from build123d import *

# Parameters (mm, degrees)
F0_R     = 47.5
F0_R_2   = 1
F1_DEPTH = 3.175


with BuildPart() as f1:
    # F0 (on Top) → F1 (new body)
    with BuildSketch(Plane.XY):
        Circle(F0_R)
        with BuildLine():
            ThreePointArc((-30.8198051534, -31.8198051534), (-32.7436846859, -32.2024885858), (-31.1126983722, -31.1126983722))
            ThreePointArc((-31.1126983722, -31.1126983722), (-30.8959256209, -31.437121721), (-30.8198051534, -31.8198051534))
        make_face(mode=Mode.SUBTRACT)
        with Locations((31.8198051534, -31.8198051534)):
            Circle(F0_R_2, mode=Mode.SUBTRACT)
        with Locations((-31.8198051534, 31.8198051534)):
            Circle(F0_R_2, mode=Mode.SUBTRACT)
        with BuildLine():
            ThreePointArc((33.3518936085, -22.0828257415), (4.0043327396, -39.7990617893), (-28.2842712475, -28.2842712475))
            ThreePointArc((-28.2842712475, -28.2842712475), (-30.9736773104, -25.3106956418), (-33.3518936085, -22.0828257415))
            ThreePointArc((-33.3518936085, -22.0828257415), (-35.0740288533, -20.25), (-35.8002348837, -17.8421742585))
            ThreePointArc((-35.8002348837, -17.8421742585), (-34.6410161514, 20), (-2.4483412752, 39.925))
            ThreePointArc((-2.4483412752, 39.925), (0, 40.5), (2.4483412752, 39.925))
            ThreePointArc((2.4483412752, 39.925), (29.1370352902, 27.4049844827), (40, 0))
            ThreePointArc((40, 0), (38.9359049936, -9.1648951072), (35.8002348837, -17.8421742585))
            ThreePointArc((35.8002348837, -17.8421742585), (35.0740288533, -20.25), (33.3518936085, -22.0828257415))
        make_face(mode=Mode.SUBTRACT)
        with Locations((31.8198051534, 31.8198051534)):
            Circle(F0_R_2, mode=Mode.SUBTRACT)
    extrude(amount=F1_DEPTH)


solid = f1.part
Design review of the part built by this model. Coordinates are the model's own, in mm. A direction names the side the tool comes from. Coordinates: 2 decimals unless noted, no trailing zeros. Order: outer loops, then holes, each group sorted by start corner. A loop starts at its lowest first (then second) coordinate and runs counter-clockwise, first axis right, second up.
Item 1: For faces 1 (the cylindrical face through (-35.056, -20.281, 1.565)), 2 (the flat face through (-11, 39, 0)), list the 3-axis set-ups (+Z, -Z, +X, -X, +Y, -Y) from which the entire face can be reached by the end or side of a thin tool; tool diameter is ignored.
Item 2: For pin 1 Ø1.5 at (x, z) = (11.5, 2) entering from -Y; pin 2 Ø1.5 at (y, z) = (6.5, 0.5) entering from -X; pin 3 Ø1.2 at (x, y) = (31.82, -31.82) entering from -Z; pin 4 Ø1.5 at (y, z) = (-33, 1.5) entering from +X, all flat-tipped, find the tip position at first contact; note any pin that passes through.
Item 3: Take a section at B-B, the plane y = 15. Write out the cut boundary in (x, z) (3 decimals).
Item 4: The part is to be moulded in two halves that separate along Y. For faces 3 (the flat face through (-11, 39, 3.175)), 4 (the cylindrical face through (0, 40.5, 1.6)), 5 (the cylindrical face through (-10.3, -46.37, 1.57)), 6 (the cylindrical face through (-34.914, 19.52, 1.565)), say which applies: pulls with the +Y half, pulls with the -Y half, needs draft (parallel to the pull), parting line crosses it, or undercut.
Item 5: For line 1 (Y direction, x = 0, z = 1); line 2 (X direction, y = 1, z = 0.5); line 3 (X direction, y = -32.5, z = 2), list the stretches that pass through material, from the lowest coordinate up.
Item 6: Take a section at A-A, the plane x = 0. Write out the cut boundary in (y, z) (3 decimals), then the cut area to 3 significant figures.
Item 7: Take a section at C-C, the plane z = 1.7. Write out the cut boundary in (x, y) (3 decimals).
The answers:
1. face 1: +Z, -Z
1. face 2: -Z, +X, -X, +Y, -Y
2. pin 1: stops at y = -46.27
2. pin 2: stops at x = -47.15
2. pin 3: passes through
2. pin 4: stops at x = 34.87
3. outline: (-45.069, 0) - (-37.081, 0) - (-37.081, 3.175) - (-45.069, 3.175) - close; (37.081, 0) - (45.069, 0) - (45.069, 3.175) - (37.081, 3.175) - close
4. face 3: needs draft
4. face 4: undercut
4. face 5: parting line crosses it
4. face 6: undercut
5. line 1: y = -47.5 to -40, 40.5 to 47.5
5. line 2: x = -47.49 to -39.99, 39.99 to 47.49
5. line 3: x = -34.64 to -32.55, -31.09 to -23.32, 23.32 to 31.09, 32.55 to 34.64
6. outline: (-47.5, 0) - (-40, 0) - (-40, 3.175) - (-47.5, 3.175) - close; (40.5, 0) - (47.5, 0) - (47.5, 3.175) - (40.5, 3.175) - close
6. area: 46.0 mm2
7. outline: circle Ø95 at (0, 0); hole (-35.8, -17.842) arc R5.5 ccw to (-33.352, -22.083) arc R40 ccw to (33.352, -22.083) arc R5.5 ccw to (35.8, -17.842) arc R40 ccw to (2.448, 39.925) arc R5.5 ccw to (-2.448, 39.925) arc R40 ccw to start; hole circle Ø2 at (-31.82, -31.82); hole circle Ø2 at (-31.82, 31.82); hole circle Ø2 at (31.82, -31.82); hole circle Ø2 at (31.82, 31.82)
